For this review, take the finished solid that the model builds, in its own axes (mm). Round coordinates to 2 decimals unless told otherwise and drop trailing zeros. Write each loop counter-clockwise with the first axis right and the second up, starting at its lowest first coordinate (ties: lowest second). Pieces come first, ordered by that corner, then holes. Notation, with made-up numbers: M 77,83.25 L 84,83.25 A18 cw 84,98.25 Z; hole C -16.5,79.5 d5. An arc over 180 degrees is marked long. Write each question's results on one line, items separated by ' | '. Start each with the question number.
```python
from build123d import *

# Parameters (mm, degrees)
SKETCH_1_W          = 200
SKETCH_1_H          = 100
EXTRUDE_1_DEPTH     = 15
SKETCH_2_R          = 5
CUT_EXTRUDE_1_DEPTH = 30
SKETCH_3_R          = 5
CUT_EXTRUDE_2_DEPTH = 30


with BuildPart() as part:
    # 草图1 → 凸台-拉伸1 (new body)
    with BuildSketch(Plane(origin=(0, 0, 0), x_dir=(1, 0, 0), z_dir=(0, 1, 0))):
        Rectangle(SKETCH_1_W, SKETCH_1_H)
    extrude(amount=EXTRUDE_1_DEPTH)

    # 草图2 → 切除-拉伸1 (cut)
    with BuildSketch(Plane(origin=(0, 0, 0), x_dir=(1, 0, 0), z_dir=(0, 1, 0))):
        with Locations(Location((-80, -30, 0), (0, 0, 90))):
            Circle(SKETCH_2_R)
        with Locations(Location((80, -30, 0), (0, 0, 90))):
            Circle(SKETCH_2_R)
        with Locations(Location((-80, 30, 0), (0, 0, 90))):
            Circle(SKETCH_2_R)
    extrude(amount=CUT_EXTRUDE_1_DEPTH, mode=Mode.SUBTRACT)

    # 草图3 → 切除-拉伸2 (cut)
    with BuildSketch(Plane(origin=(0, 0, 0), x_dir=(1, 0, 0), z_dir=(0, 1, 0))):
        with Locations(Location((80, 30, 0), (0, 0, 90))):
            Circle(SKETCH_3_R)
    extrude(amount=CUT_EXTRUDE_2_DEPTH, mode=Mode.SUBTRACT)


solid = part.part
```
Item 1: We need section C-C on y = 8.5. State the section outline as (x, z) points.
Item 2: For probe 1 along X at (y, z) = (11.5, -30); probe 2 along Z at (x, y) = (80, 3); probe 3 along X at (y, z) = (3.5, -31.5), list the stretches that pass through material, from the lowest coordinate up.
Item 3: We need section B-B on z = -30. State the section outline as (x, y) points, then the cut area to 3 significant figures.
Item 4: We need section A-A on x = -80. State the section outline as (y, z) points, then the cut area to 3 significant figures.
Item 5: Mouldability with a two-part tool opening along X and no side actions: class faces 1 (the flat face through (-100, 7, 1)), 2 (the flat face through (100, 7, 1)), 3 (the flat face through (-1, 7, 50)), 4 (the cylindrical face through (84.88, 7.4, 31.08)) as pulls with the +X half, pulls with the -X half, needs draft (parallel to the pull), parting line crosses it, or undercut.
Numbers:
1) outline: M -100,-50 L 100,-50 L 100,50 L -100,50 Z; hole C -80,-30 d10; hole C -80,30 d10; hole C 80,-30 d10; hole C 80,30 d10
2) probe 1: x = -100 to -85, -75 to 75, 85 to 100 | probe 2: z = -50 to -35, -25 to 25, 35 to 50 | probe 3: x = -100 to -84.77, -75.23 to 75.23, 84.77 to 100
3) outline: M -100,0 L -85,0 L -85,15 L -100,15 Z; M -75,0 L 75,0 L 75,15 L -75,15 Z; M 85,0 L 100,0 L 100,15 L 85,15 Z | area: 2,700 mm^2
4) outline: M 0,-50 L 15,-50 L 15,-35 L 0,-35 Z; M 0,-25 L 15,-25 L 15,25 L 0,25 Z; M 0,35 L 15,35 L 15,50 L 0,50 Z | area: 1,200 mm^2
5) face 1: pulls with the -X half | face 2: pulls with the +X half | face 3: needs draft | face 4: undercut
